from build123d import *

# Parameters (mm, degrees)
BOSS_EXTRU_1_OUTLINE_W   = 55
BOSS_EXTRU_1_OUTLINE_H   = 47
BOSS_EXTRU_1_OUTLINE_W_2 = 5
BOSS_EXTRU_1_OUTLINE_H_2 = 5
BOSS_EXTRU_1_OUTLINE_R   = 1.5
BOSS_EXTRU_1_OUTLINE_R_2 = 2.5
BOSS_EXTRU_1_DEPTH       = 6
CONG_1_R                 = 4


# Read off the part's stored shape, not the designer's step: Boss.-Extru.1
with BuildPart() as part:
    # Boss.-Extru.1 outline → Boss.-Extru.1 (new body)
    with BuildSketch(Plane.XY):
        Rectangle(BOSS_EXTRU_1_OUTLINE_W, BOSS_EXTRU_1_OUTLINE_H)
        with Locations((-20, -16)):
            Rectangle(BOSS_EXTRU_1_OUTLINE_W_2, BOSS_EXTRU_1_OUTLINE_H_2, mode=Mode.SUBTRACT)
        with Locations((-12.5, -16)):
            Circle(BOSS_EXTRU_1_OUTLINE_R, mode=Mode.SUBTRACT)
        with Locations((-5, -16)):
            Rectangle(BOSS_EXTRU_1_OUTLINE_W_2, BOSS_EXTRU_1_OUTLINE_H_2, mode=Mode.SUBTRACT)
        with Locations((5, -16)):
            Rectangle(BOSS_EXTRU_1_OUTLINE_W_2, BOSS_EXTRU_1_OUTLINE_H_2, mode=Mode.SUBTRACT)
        with Locations((12.5, -16)):
            Circle(BOSS_EXTRU_1_OUTLINE_R, mode=Mode.SUBTRACT)
        with Locations((20, -16)):
            Rectangle(BOSS_EXTRU_1_OUTLINE_W_2, BOSS_EXTRU_1_OUTLINE_H_2, mode=Mode.SUBTRACT)
        with Locations((-20, 16)):
            Rectangle(BOSS_EXTRU_1_OUTLINE_W_2, BOSS_EXTRU_1_OUTLINE_H_2, mode=Mode.SUBTRACT)
        with Locations((-12.5, 16)):
            Circle(BOSS_EXTRU_1_OUTLINE_R, mode=Mode.SUBTRACT)
        with Locations((-5, 16)):
            Rectangle(BOSS_EXTRU_1_OUTLINE_W_2, BOSS_EXTRU_1_OUTLINE_H_2, mode=Mode.SUBTRACT)
        Circle(BOSS_EXTRU_1_OUTLINE_R_2, mode=Mode.SUBTRACT)
        with Locations((5, 16)):
            Rectangle(BOSS_EXTRU_1_OUTLINE_W_2, BOSS_EXTRU_1_OUTLINE_H_2, mode=Mode.SUBTRACT)
        with Locations((12.5, 16)):
            Circle(BOSS_EXTRU_1_OUTLINE_R, mode=Mode.SUBTRACT)
        with Locations((20, 16)):
            Rectangle(BOSS_EXTRU_1_OUTLINE_W_2, BOSS_EXTRU_1_OUTLINE_H_2, mode=Mode.SUBTRACT)
    extrude(amount=BOSS_EXTRU_1_DEPTH)

    # Congé1
    cong_1_edges = [part.edges().sort_by_distance(p)[0] for p in [
        (-27.5, 23.5, 3),
        (27.5, 23.5, 3),
        (27.5, -23.5, 3),
        (-27.5, -23.5, 3),
    ]]
    fillet(cong_1_edges, radius=CONG_1_R)


solid = part.part
Geometry check sheet. Reference: the model listing, model coordinates, mm. A direction names the side the tool comes from. Coordinates: 2 decimals unless noted, no trailing zeros. Order: outer loops, then holes, each group sorted by start corner. A loop starts at its lowest first (then second) coordinate and runs counter-clockwise, first axis right, second up. Notation, with made-up numbers: (51, 63) - (60, 63) arc R23 cw to (60, 83) - close; hole circle Ø4 at (-28.75, 35.25). An arc over 180 degrees is marked (long way). One line per item, written item: value.
(1) Sectioned sample at B-B (y = 0). Enter the section's corners in (x, z), and give its area (3 significant figures).
Data:
outline: (-27.5, 0) - (-2.5, 0) - (-2.5, 6) - (-27.5, 6) - close; (2.5, 0) - (27.5, 0) - (27.5, 6) - (2.5, 6) - close
area: 300 mm^2
(2) Depth check by flat-ended pin: pin 1 Ø2.5 at (x, y) = (-12.5, -16) entering from +Z. Enter the tip coordinate at first touch or a pass-through.
Data:
pin 1: passes through
(3) Thickness scan on probe 1 along Y at (x, z) = (3.5, 2.4); probe 2 along Y at (x, z) = (12.5, 2.95); probe 3 along X at (y, z) = (14, 2.35). Record the ranges inside material, lowest first. Write a range as from..to.
Data:
probe 1: y = -23.5..-18.5, -13.5..13.5, 18.5..23.5
probe 2: y = -23.5..-17.5, -14.5..14.5, 17.5..23.5
probe 3: x = -27.5..-22.5, -17.5..-7.5, -2.5..2.5, 7.5..17.5, 22.5..27.5
(4) Sectioned sample at D-D (y = 16). Enter the section's corners in (x, z).
Data:
outline: (-27.5, 0) - (-22.5, 0) - (-22.5, 6) - (-27.5, 6) - close; (-17.5, 0) - (-14, 0) - (-14, 6) - (-17.5, 6) - close; (-11, 0) - (-7.5, 0) - (-7.5, 6) - (-11, 6) - close; (-2.5, 0) - (2.5, 0) - (2.5, 6) - (-2.5, 6) - close; (7.5, 0) - (11, 0) - (11, 6) - (7.5, 6) - close; (14, 0) - (17.5, 0) - (17.5, 6) - (14, 6) - close; (22.5, 0) - (27.5, 0) - (27.5, 6) - (22.5, 6) - close
(5) Sectioned sample at A-A (x = 0). Enter the section's corners in (y, z), and give its area (3 significant figures).
Data:
outline: (-23.5, 0) - (-2.5, 0) - (-2.5, 6) - (-23.5, 6) - close; (2.5, 0) - (23.5, 0) - (23.5, 6) - (2.5, 6) - close
area: 252 mm^2
(6) Sectioned sample at C-C (x = -21). Enter the section's corners in (y, z), and give its area (3 significant figures).
Data:
outline: (-23.5, 0) - (-18.5, 0) - (-18.5, 6) - (-23.5, 6) - close; (-13.5, 0) - (13.5, 0) - (13.5, 6) - (-13.5, 6) - close; (18.5, 0) - (23.5, 0) - (23.5, 6) - (18.5, 6) - close
area: 222 mm^2
(7) Release check for a two-part mould opening along Y. For faces 3 (the face through (11, -16, 3)), 4 (the face through (-14, -16, 3)), 5 (the face through (0, 6, 0)), 6 (the face through (26.297, -22.359, 3.042)) record: +Y half, -Y half, draft (parallel to the pull), parting line (faces both ways), or undercut.
Data:
face 3: undercut
face 4: undercut
face 5: draft
face 6: -Y half
(8) Access from +Z, -Z, +X, -X, +Y, -Y to the whole of each face (thin tool, end or side, straight path). Record for faces 1 (the face through (-27.5, 0, 3)), 2 (the face through (-2.5, -16, 3)).
Data:
face 1: +Z, -Z, -X, +Y, -Y
face 2: +Z, -Z
